Part model, mm, in its own coordinate system. Give positions to 0.01 mm unless a question says otherwise; leave off trailing zeros. Order: outer loops, then holes, each group sorted by start corner. A loop starts at its lowest first (then second) coordinate and runs counter-clockwise, first axis right, second up. Notation, with made-up numbers: (56, 54.5) - (63, 54.5) arc R28 cw to (63, 73.5) - close; hole circle Ø11 at (-19, 40). An arc over 180 degrees is marked (long way). One line per item, written item: value.
```python
from build123d import *

# Parameters (mm, degrees)
BOSS_EXTRUDE1_DEPTH        = 3
SKETCH2_W                  = 50
SKETCH2_H                  = 50
CUT_EXTRUDE1_DEPTH         = 10
SKETCH3_W                  = 3
SKETCH3_H                  = 480
BOSS_EXTRUDE2_DEPTH        = 20
SKETCH5_W                  = 3
SKETCH5_H                  = 400
BOSS_EXTRUDE3_DEPTH        = 25
SKETCH6_W                  = 3
SKETCH6_H                  = 402.54833996
BOSS_EXTRUDE4_DEPTH        = 25
SKETCH7_W                  = 25.200898878
SKETCH7_H                  = 14.317309472
CUT_EXTRUDE2_DEPTH         = 25
F_3_2_3_2_DIAMETER_HOLE1_D = 3.2
F_5_5_5_5_DIAMETER_HOLE1_D = 5.5


with BuildPart() as part:
    # Sketch1 → Boss-Extrude1 (new body)
    with BuildSketch(Plane(origin=(0, 0, 0), x_dir=(0, 0, -1), z_dir=(1, 0, 0))):
        Polygon((31.669668796, 625.573683549), (191.669668796, 173.025343589), (-258.330331204, 173.025343589), (-258.330331204, 625.573683549), align=None)
    extrude(amount=BOSS_EXTRUDE1_DEPTH)

    # Sketch2 → Cut-Extrude1 (cut)
    with BuildSketch(Plane.ZY):
        with Locations((233.330331204, 198.025343589)):
            Rectangle(SKETCH2_W, SKETCH2_H)
    extrude(amount=-CUT_EXTRUDE1_DEPTH, mode=Mode.SUBTRACT)

    # Sketch3 → Boss-Extrude2 (add)
    with BuildSketch(Plane(origin=(0, 79.461003756, -224.749658383), x_dir=(-1, 0, 0), z_dir=(0, 0.3333333333333335, -0.9428090415820635))):
        with Locations((-1.5, 339.23996876)):
            Rectangle(SKETCH3_W, SKETCH3_H)
    extrude(amount=BOSS_EXTRUDE2_DEPTH)

    # Sketch5 → Boss-Extrude3 (add)
    with BuildSketch(Plane.XZ.offset(-173.025343589)):
        with Locations((1.5, 8.330331204)):
            Rectangle(SKETCH5_W, SKETCH5_H)
    extrude(amount=BOSS_EXTRUDE3_DEPTH)

    # Sketch6 → Boss-Extrude4 (add)
    with BuildSketch(Plane.XY.offset(258.330331204)):
        with Locations((1.5, 424.299513569)):
            Rectangle(SKETCH6_W, SKETCH6_H)
    extrude(amount=BOSS_EXTRUDE4_DEPTH)

    # Sketch7 → Cut-Extrude2 (cut)
    with BuildSketch(Plane(origin=(3, 0, 0), x_dir=(0, 0, -1), z_dir=(1, 0, 0))):
        with Locations((44.270118235, 632.732338285)):
            Rectangle(SKETCH7_W, SKETCH7_H)
    extrude(amount=-CUT_EXTRUDE2_DEPTH, mode=Mode.SUBTRACT)

    # Ø3.2 (3.2) Diameter Hole1 (through all)
    with Locations(Plane(origin=(3, 0, 0), x_dir=(0, 0, -1), z_dir=(1, 0, 0))):
        with Locations((191.097759212, 204.64294817), (156.097759212, 303.637897536), (121.097759212, 402.632846902), (86.097759212, 501.627796268), (51.097759212, 600.622745635)):
            Hole(F_3_2_3_2_DIAMETER_HOLE1_D / 2)

    # Ø5.5 (5.5) Diameter Hole1 (through all)
    with Locations(Plane(origin=(3, 0, 0), x_dir=(0, 0, -1), z_dir=(1, 0, 0))):
        with Locations((161.669668796, 158.025343589), (76.669668796, 158.025343589), (-8.330331204, 158.025343589), (-93.330331204, 158.025343589), (-178.330331204, 158.025343589), (-273.330331204, 253.025343589), (-273.330331204, 333.025343589), (-273.330331204, 413.025343589), (-273.330331204, 493.025343589), (-273.330331204, 573.025343589)):
            Hole(F_5_5_5_5_DIAMETER_HOLE1_D / 2)


solid = part.part
```
1) Slice it at C-C on y = 347. Write the cut outline in (x, z), then the cut area to 3 significant figures.
Answer:
outline: (0, -151.37) - (3, -151.37) - (3, 283.33) - (0, 283.33) - close
area: 1,300 mm2
2) Drop flat-ended pins along their axis: P1, Ø1.5, axis at x = 2, z = 240.5, coming from the -Y side; P2, Ø1.5, axis at x = 1.5, y = 162, coming from the -Z side; P3, Ø0.9, axis at x = 2, y = 175.5, coming from the +Z side. Give the stop position or say it passes through.
Answer:
P1: stops at y = 223.03
P2: stops at z = -191.67
P3: stops at z = 208.33
3) Wall check: line 1 along Z through (x, y) = (2.3, 253.5); line 2 along Y through (x, z) = (0.5, 234.5); line 3 along Z through (x, y) = (1.8, 551). Give the ranges that are in metal, low to high. Write a range as [from, to].
Answer:
line 1: z = [-184.43, 270.62], [276.04, 283.33]
line 2: y = [223.03, 625.57]
line 3: z = [-79.25, 283.33]
4) Slice it at B-B on z = -147.5. Write the cut outline in (x, y).
Answer:
outline: (0, 148.03) - (3, 148.03) - (3, 357.96) - (0, 357.96) - close
5) Slice it at A-A on x = 1.85. Count the separate pieces of the cut face and the enclosed holes in it, then the cut area to 3 significant figures.
Answer:
separate pieces: 1
enclosed holes: 15
area: 194,000 mm2
